from build123d import *

# Parameters (mm, degrees)
SKETCH1_W           = 102
SKETCH1_H           = 35
BOSS_EXTRUDE1_DEPTH = 8.7
BOSS_EXTRUDE2_DEPTH = 102
SKETCH5_R           = 3.5
BOSS_EXTRUDE3_DEPTH = 20


with BuildPart() as part:
    # Sketch1 → Boss-Extrude1 (new body)
    with BuildSketch(Plane.XY):
        Rectangle(SKETCH1_W, SKETCH1_H)
    extrude(amount=BOSS_EXTRUDE1_DEPTH)

    # Sketch4 → Boss-Extrude2 (add)
    with BuildSketch(Plane.ZY.offset(51)):
        Polygon((6.5, -17.5), (8.7, -17.5), (8.7, -20.045584412), (3.954415588, -20.045584412), align=None)
    extrude(amount=-BOSS_EXTRUDE2_DEPTH)

    # Sketch5 → Boss-Extrude3 (add)
    with BuildSketch(Plane(origin=(0, 0, 0), x_dir=(-1, 0, 0), z_dir=(0, 0, -1))):
        with Locations((-39.57, 10.64)):
            Circle(SKETCH5_R)
        with Locations((-14.17, 10.64)):
            Circle(SKETCH5_R)
        with Locations((11.23, 10.64)):
            Circle(SKETCH5_R)
        with Locations((36.63, 10.64)):
            Circle(SKETCH5_R)
    extrude(amount=BOSS_EXTRUDE3_DEPTH)


solid = part.part
The listing builds one solid part. Answer for the finished solid, in the listing's coordinates (mm). A direction names the side the tool comes from. Give positions to 0.01 mm unless a question says otherwise; leave off trailing zeros. Write each loop counter-clockwise with the first axis right and the second up, starting at its lowest first coordinate (ties: lowest second). Pieces come first, ordered by that corner, then holes. Notation, with made-up numbers: (67.25, 17) -> (122.25, 17) arc R17 cw to (122.25, 50) -> close; hole circle Ø10 at (-34, 55). An arc over 180 degrees is marked (long way). One line per question, with ' | ' between items. Start each with the question number.
1. Given pin 1 Ø3 at (y, z) = (9.5, -13.5) entering from -X; pin 2 Ø1 at (y, z) = (8, -1) entering from -X; pin 3 Ø3 at (x, z) = (40, -6) entering from +Y, each flat-ended and moving along its own axis, determine where each tip first touches the part or whether it passes through.
2. For faces 1 (the flat face through (-1, -20.046, 6)), 2 (the cylindrical face through (36.337, 9.299, -9.86)), determine the directions among +Z, -Z, +X, -X, +Y, -Y from which every point of the face is accessible in a straight line to the end or side of a thin tool.
3. Section C-C (y = 10.64) is taken. Determine the outline of the cut face in (x, z), plus the area to 3 significant figures.
4. Find the intervals of material crossed by probe 1 along X at (y, z) = (11, -1.5); probe 2 along X at (y, z) = (13, -9.75); probe 3 along Z at (x, y) = (17.5, -10.5), in increasing order.
5. Section B-B (z = -8.5) is taken. Determine the outline of the cut face in (x, y).
6. Section D-D (x = -23.5) is taken. Determine the outline of the cut face in (y, z).
7. Section A-A (x = -11.23) is taken. Determine the outline of the cut face in (y, z), plus the area to 3 significant figures.
8. For a pull along X with two mould halves and no side action, classify faces 3 (the flat face through (51, -1, 4)), 4 (the flat face through (14, 11, -20)), 5 (the cylindrical face through (-7.733, 10.794, -9.86)) as pulls with the +X half, pulls with the -X half, needs draft (parallel to the pull), parting line crosses it, or undercut.
Response values:
1) pin 1: x = -40.13 | pin 2: x = -39.4 | pin 3: y = 14.14
2) face 1: +Z, -Z, +X, -X, -Y | face 2: -Z
3) outline: (-51, 0) -> (-40.13, 0) -> (-40.13, -20) -> (-33.13, -20) -> (-33.13, 0) -> (-14.73, 0) -> (-14.73, -20) -> (-7.73, -20) -> (-7.73, 0) -> (10.67, 0) -> (10.67, -20) -> (17.67, -20) -> (17.67, 0) -> (36.07, 0) -> (36.07, -20) -> (43.07, -20) -> (43.07, 0) -> (51, 0) -> (51, 8.7) -> (-51, 8.7) -> close | area: 1,450 mm2
4) probe 1: -40.11 to -33.15, -14.71 to -7.75, 10.69 to 17.65, 36.09 to 43.05 | probe 2: -39.21 to -34.05, -13.81 to -8.65, 11.59 to 16.75, 36.99 to 42.15 | probe 3: 0 to 8.7
5) outline: circle Ø7 at (-36.63, 10.64); circle Ø7 at (-11.23, 10.64); circle Ø7 at (14.17, 10.64); circle Ø7 at (39.57, 10.64)
6) outline: (-20.05, 3.95) -> (-17.5, 6.5) -> (-17.5, 0) -> (17.5, 0) -> (17.5, 8.7) -> (-20.05, 8.7) -> close
7) outline: (-20.05, 3.95) -> (-17.5, 6.5) -> (-17.5, 0) -> (7.14, 0) -> (7.14, -20) -> (14.14, -20) -> (14.14, 0) -> (17.5, 0) -> (17.5, 8.7) -> (-20.05, 8.7) -> close | area: 453 mm2
8) face 3: pulls with the +X half | face 4: needs draft | face 5: undercut
